For this review, take the finished solid that the model builds, in its own axes (mm). A direction names the side the tool comes from. Give positions to 0.01 mm unless a question says otherwise; leave off trailing zeros. Loops run counter-clockwise (first coordinate to the right, second up) from the corner with the lowest first, then second, coordinate; pieces in that order, holes last. Notation, with made-up numbers: (13, 78.25) - (18, 78.25) arc R28 ccw to (18, 106.25) - close; hole circle Ø9 at (43.5, 25). An arc over 180 degrees is marked (long way). Put each result on its own line as item: value.
Autodesk Inventor part; units mm, degrees
ref_plane "YZ Plane" through (0, 0, 0) normal (1, 0, 0) x (0, 1, 0)
ref_plane "XZ Plane" through (0, 0, 0) normal (0, 1, 0) x (-1, 0, 0)
ref_plane "XY Plane" through (0, 0, 0) normal (0, 0, 1) x (1, 0, 0)
sketch "Sketch1" plane through (0, 0, 0) normal (0, 0, 1) x (1, 0, 0)
  line L0 (215.9, -165.1) -> (-215.9, -165.1)
  line L1 (-215.9, -165.1) -> (-215.9, 165.1)
  line L2 (215.9, 165.1) -> (215.9, -165.1)
  line L3 (215.9, -165.1) -> (-215.9, 165.1) construction
  line L4 (-215.9, -165.1) -> (215.9, 165.1) construction
  line L5 (76.2, 101.6) -> (-76.4881, 101.6)
  line L6 (-76.2, 191.0151) -> (76.2, 101.6) construction
  line L7 (76.2, 191.0151) -> (-76.4881, 101.6) construction
  line L8 (66.0896, 101.6) -> (-66.0896, 101.6)
  line L9 (-67.8456, 164.5323) -> (67.5575, 164.5323)
  line L10 (76.2, 139.1323) -> (-76.4881, 139.1323)
  line L11 (-76.4881, 155.8898) -> (-67.8456, 164.5323)
  line L12 (-0.144, 139.1323) -> (-0.144, 146.3921)
  line L13 (76.2, 155.8898) -> (67.5575, 164.5323)
  line L14 (-215.9, 165.1) -> (-85.6983, 165.1)
  line L15 (-67.8456, 164.5323) -> (67.5575, 164.5323)
  line L16 (85.4102, 165.1) -> (215.9, 165.1)
  line L17 (76.2, 139.1323) -> (76.2, 101.6)
  line L18 (-76.4881, 101.6) -> (-76.4881, 139.1323)
  line L19 (-76.4881, 155.8898) -> (-85.6983, 165.1)
  line L20 (76.2, 155.8898) -> (85.4102, 165.1)
  point P0 (0, 0)
  point P1 (-0.072, 146.3498)
  dimension "d0" = 431.8
  dimension "d1" = 330.2
  dimension "d7" = 266.7
  dimension "d11" = 25.4
  dimension "d12" = 45
extrude "Extrusion1" add sketch "Sketch1" along normal blind 85.725
chamfer "Chamfer1" distance 25.4 angle 45 4 edges at (215.9, 165.1, 42.8625) (215.9, -165.1, 42.8625) (-215.9, -165.1, 42.8625) (-215.9, 165.1, 42.8625)
sketch "Sketch2" plane through (0, 0, 85.725) normal (0, 0, 1) x (1, 0, 0)
  line L0 (76.2, 139.1323) -> (76.2, 101.6)
  line L1 (76.2, 101.6) -> (-76.4881, 101.6)
  line L2 (-76.4881, 101.6) -> (-76.4881, 139.1323)
  line L3 (-215.9, 139.7) -> (-190.5, 165.1)
  line L4 (-215.9, 139.7) -> (-215.9, -139.7)
  line L5 (-190.5, -165.1) -> (-215.9, -139.7)
  line L6 (-190.5, -165.1) -> (190.5, -165.1)
  line L7 (215.9, -139.7) -> (190.5, -165.1)
  line L8 (215.9, -139.7) -> (215.9, 139.7)
  line L9 (190.5, 165.1) -> (215.9, 139.7)
  line L10 (190.5, 165.1) -> (85.4102, 165.1)
  line L11 (85.4102, 165.1) -> (76.2, 155.8898)
  line L12 (76.2, 155.8898) -> (67.5575, 164.5323)
  line L13 (67.5575, 164.5323) -> (-67.8456, 164.5323)
  line L14 (-67.8456, 164.5323) -> (-76.4881, 155.8898)
  line L15 (-76.4881, 155.8898) -> (-85.6983, 165.1)
  line L16 (-85.6983, 165.1) -> (-190.5, 165.1)
  line L17 (-76.4881, 139.1323) -> (76.2, 139.1323)
  line L18 (-76.4881, 139.1323) -> (-76.4881, 155.8898)
  line L19 (76.2, 139.1323) -> (76.2, 155.8898)
  point P0 (0, 0)
extrude "Extrusion2" cut sketch "Sketch2" against normal blind 30.1625 contours L17 L18 L14 L13 L12 L19
sketch "Sketch3" plane through (0, 0, 0) normal (0, 0, -1) x (-1, 0, 0)
  line L0 (76.4881, 139.1323) -> (76.4881, 101.6)
  line L1 (76.4881, 101.6) -> (-76.2, 101.6)
  line L2 (-76.2, 101.6) -> (-76.2, 139.1323)
  line L3 (-76.2, 139.1323) -> (76.4881, 139.1323)
  line L4 (190.5, 165.1) -> (215.9, 139.7)
  line L5 (85.6983, 165.1) -> (190.5, 165.1)
  line L6 (76.4881, 155.8898) -> (85.6983, 165.1)
  line L7 (67.8456, 164.5323) -> (76.4881, 155.8898)
  line L8 (-67.5575, 164.5323) -> (67.8456, 164.5323)
  line L9 (-76.2, 155.8898) -> (-67.5575, 164.5323)
  line L10 (-85.4102, 165.1) -> (-76.2, 155.8898)
  line L11 (-190.5, 165.1) -> (-85.4102, 165.1)
  line L12 (-215.9, 139.7) -> (-190.5, 165.1)
  line L13 (-215.9, -139.7) -> (-215.9, 139.7)
  line L14 (-190.5, -165.1) -> (-215.9, -139.7)
  line L15 (190.5, -165.1) -> (-190.5, -165.1)
  line L16 (215.9, -139.7) -> (190.5, -165.1)
  line L17 (215.9, 139.7) -> (215.9, -139.7)
  line L18 (-76.2, 139.1323) -> (76.4881, 139.1323)
  line L19 (-76.2, 139.1323) -> (-76.2, 155.8898)
  line L20 (76.4881, 101.6) -> (76.4881, 155.8898)
  line L21 (76.4881, 139.1323) -> (76.4881, 155.8898)
  point P0 (0, 0)
extrude "Extrusion3" cut sketch "Sketch3" against normal blind 30.1625 contours L3 L19 L9 L8 L7 L20
chamfer "Chamfer2" distance 3.175 angle 45 4 edges at (-0.144, 139.1323, 55.5625) (-0.144, 139.1323, 30.1625) (-0.144, 164.5323, 55.5625) (-0.144, 164.5323, 30.1625)
properties part number "Divider_box"
1) Draft analysis for pull direction Y (two halves, no side actions). For faces 4 (the face through (-203, 152.6, 42.3)), 5 (the face through (-76.488, 128, 42)), 6 (the face through (203.4, -152.2, 43.5)), state which applies: pulls with the +Y half, pulls with the -Y half, needs draft (parallel to the pull), parting line crosses it, or undercut.
Geometry check:
face 4: pulls with the +Y half
face 5: undercut
face 6: pulls with the -Y half
2) Wall thickness on line 1 (Y direction, x = -12, z = 51); line 2 (Y direction, x = 16.5, z = 57); line 3 (Y direction, x = 80.5, z = 56.5): over which ranges is each line inside the solid? List them lowest first.
Geometry check:
line 1: y = -165.1 to 101.6, 139.13 to 164.53
line 2: y = -165.1 to 101.6
line 3: y = -165.1 to 160.19
3) Take a section at C-C on z = 7. State the section outline as (x, y) points, and give its area (3 significant figures).
Geometry check:
outline: (-215.9, -139.7) - (-190.5, -165.1) - (190.5, -165.1) - (215.9, -139.7) - (215.9, 139.7) - (190.5, 165.1) - (85.41, 165.1) - (76.2, 155.89) - (76.2, 101.6) - (-76.49, 101.6) - (-76.49, 155.89) - (-85.7, 165.1) - (-190.5, 165.1) - (-215.9, 139.7) - close
area: 132,000 mm²
4) For faces 1 (the face through (1, 101.6, 42)), 2 (the face through (76.2, 129, 42)), 3 (the face through (80.74, 160.43, 42.26)), list the 3-axis set-ups (+Z, -Z, +X, -X, +Y, -Y) from which the entire face can be reached by the end or side of a thin tool; tool diameter is ignored.
Geometry check:
face 1: +Z, -Z
face 2: none
face 3: +Z, -Z, +Y
5) Take a section at B-B on x = 38.5. State the section outline as (y, z) points (1 decimal).
Geometry check:
outline: (-165.1, 0) - (101.6, 0) - (101.6, 85.7) - (-165.1, 85.7) - close; (139.1, 33.3) - (142.3, 30.2) - (161.4, 30.2) - (164.5, 33.3) - (164.5, 52.4) - (161.4, 55.6) - (142.3, 55.6) - (139.1, 52.4) - close
6) Insertion check: pin 1 Ø2 at (x, y) = (-88.5, 104) entering from -Z; pin 2 Ø5.5 at (x, z) = (-8, 43.5) entering from +Y; pin 3 Ø15 at (x, y) = (-33.5, 149.5) entering from -Z; pin 4 Ø9.5 at (x, y) = (-0.5, 149) entering from +Z. Each pin has a flat end and moves straight along its axis. Give the tip position at first contact, or say it passes through.
Geometry check:
pin 1: stops at z = 0
pin 2: stops at y = 164.53
pin 3: stops at z = 30.16
pin 4: stops at z = 55.56
7) Take a section at A-A on z = 47.5. State the section outline as (x, y) points, and give its area (3 significant figures).
Geometry check:
outline: (-215.9, -139.7) - (-190.5, -165.1) - (190.5, -165.1) - (215.9, -139.7) - (215.9, 139.7) - (190.5, 165.1) - (85.41, 165.1) - (76.2, 155.89) - (67.56, 164.53) - (-67.85, 164.53) - (-76.49, 155.89) - (-85.7, 165.1) - (-190.5, 165.1) - (-215.9, 139.7) - close; hole (-76.49, 101.6) - (76.2, 101.6) - (76.2, 139.13) - (-76.49, 139.13) - close
area: 135,000 mm²
